Can you work these out from the model? Positions are in its coordinate system, mm. Face numbers are marked on the shaded views. A direction names the side the tool comes from. Give positions to 0.01 mm unless a question says otherwise; leave off trailing zeros. Order: outer loops, then holes, each group sorted by start corner. A loop starts at its lowest first (then second) coordinate and runs counter-clockwise, first axis right, second up. Notation, with made-up numbers: M 34.25,29 L 50.25,29 A18 cw 50.25,56 Z; hole C 22.5,15.25 d4. An arc over 180 degrees is marked long. Use one line per item in the form item = value. Start each with the question number.
1. I want a section at D-D, the plane z = -407.5. List the corners of the cut face in (x, y) for me, and give its area (3 significant figures).
2. I want a section at B-B, the plane x = -337.5. List the corners of the cut face in (y, z) for me, and give its area (3 significant figures).
3. I want a section at A-A, the plane z = -257. List the corners of the cut face in (x, y) for me, and give its area (3 significant figures).
4. We'd pull the mould along Y, two halves only. Please class the marked faces 1, 2 and 3: +Y half, -Y half, draft (parallel to the pull), parting line (faces both ways), or undercut.
5. Will these pins go through, and if not, where does the flat tip stop? P1, Ø7, axis at y = -237, z = -459, coming from the +X side; P2, Ø12, axis at x = 105.5, z = -649.5, coming from the +Y side; P3, Ø4, axis at y = -147, z = -600.5, coming from the +X side; P4, Ø6, axis at x = 309, y = -69, coming from the +Z side.
6. For the marked faces 4, 5 and 6, which set-ups out of +Z, -Z, +X, -X, +Y, -Y let a thin tool reach every point of the face, with its end or its side?
7. I need wall thicknesses on L1, parallel to Y at x = -5.5, z = -684.5; L2, parallel to Y at x = 99, z = -420.5; L3, parallel to X at y = 13, z = -487.5. Which ranges of each line are inside material? Lowest first, please.
```python
from build123d import *

# Parameters (mm, degrees)
F0_W      = 76.2
F0_H      = 76.2
F1_DEPTH  = 812.8
F2_DEPTH  = 736.6
F0_W_2    = 800.1
F0_H_2    = 482.6
F3_DEPTH  = 25.4
F4_W      = 355.6
F4_H      = 76.2
F5_DEPTH  = 101.6
F6_R      = 38.09999
F7_W      = 298.45
F7_H      = 533.4
F7_W_2    = 12.7
F7_H_2    = 127
F7_W_3    = 622.3
F7_H_3    = 101.6
F7_W_4    = 127
F7_H_4    = 12.7
F8_DEPTH  = 6.35
F9_DEPTH  = 12.7
F10_W     = 222.25
F10_H     = 482.6
F11_DEPTH = 25.4
F12_W     = 622.3
F12_H     = 304.8
F13_DEPTH = 635


# Not quite as in the source:
# - a fillet or chamfer is up to 0.001 mm smaller than in the source, because OpenCascade refuses the exact size


with BuildPart() as f1:
    # F0 (on Top) → F1 (new body)
    with BuildSketch(Plane.XY):
        with Locations((-349.25, 190.5)):
            Rectangle(F0_W, F0_H)
    extrude(amount=-F1_DEPTH)



with BuildPart() as f1b:
    # F0 (on Top) → F1, piece 2 (new body)
    with BuildSketch(Plane.XY):
        with Locations((-349.25, -190.5)):
            Rectangle(F0_W, F0_H)
    extrude(amount=-F1_DEPTH)


with BuildPart() as f1c:
    # F0 (on Top) → F1, piece 3 (new body)
    with BuildSketch(Plane.XY):
        with Locations((349.25, -190.5)):
            Rectangle(F0_W, F0_H)
    extrude(amount=-F1_DEPTH)


with BuildPart() as f1d:
    # F0 (on Top) → F1, piece 4 (new body)
    with BuildSketch(Plane.XY):
        with Locations((349.25, 190.5)):
            Rectangle(F0_W, F0_H)
    extrude(amount=-F1_DEPTH)


with BuildPart() as f1_1:
    add(f1.part)

    add(f1b.part)  # F2 merges F1b

    add(f1c.part)  # F2 merges F1c

    add(f1d.part)  # F2 merges F1d
    # F0 (on Top) → F2 (join)
    with BuildSketch(Plane.XY):
        with Locations((-349.25, 190.5)):
            Rectangle(F0_W, F0_H)
        Polygon((311.15, 152.4), (311.15, 228.6), (-311.15, 228.6), (-311.15, 152.4), (-387.35, 152.4), (-387.35, -152.4), (-311.15, -152.4), (-311.15, -228.6), (311.15, -228.6), (311.15, -152.4), (387.35, -152.4), (387.35, 152.4), align=None)
        with Locations((-349.25, -190.5)):
            Rectangle(F0_W, F0_H)
        with Locations((349.25, -190.5)):
            Rectangle(F0_W, F0_H)
        with Locations((349.25, 190.5)):
            Rectangle(F0_W, F0_H)
    extrude(amount=-F2_DEPTH)

    # F0 (on Top) → F3 (join)
    with BuildSketch(Plane.XY):
        Rectangle(F0_W_2, F0_H_2)
        Polygon((311.15, 228.6), (387.35, 228.6), (387.35, 152.4), (387.35, -152.4), (387.35, -228.6), (311.15, -228.6), (-311.15, -228.6), (-387.35, -228.6), (-387.35, -152.4), (-387.35, 152.4), (-387.35, 228.6), (-311.15, 228.6), align=None, mode=Mode.SUBTRACT)
    extrude(amount=-F3_DEPTH)

    # F4 (on face) → F5 (join)
    with BuildSketch(Plane.YZ.offset(387.35)):
        with Locations((0, -139.7)):
            Rectangle(F4_W, F4_H)
    extrude(amount=F5_DEPTH)

    # F6 (radius 38.1 in the source; OpenCascade refuses exactly that, so slightly less here)
    f6_edges = [f1_1.edges().sort_by_distance(p)[0] for p in [
        (488.95, 0, -101.6),
        (488.95, 0, -177.8),
    ]]
    fillet(f6_edges, radius=F6_R)

    # F7 (on face) → F8 (join)
    with BuildSketch(Plane.XZ.offset(228.6)):
        with Locations((161.925, -444.5)):
            Rectangle(F7_W, F7_H)
        with Locations((44.45, -444.5)):
            Rectangle(F7_W_2, F7_H_2, mode=Mode.SUBTRACT)
        with Locations((-161.925, -444.5)):
            Rectangle(F7_W, F7_H)
        with Locations((-44.45, -444.5)):
            Rectangle(F7_W_2, F7_H_2, mode=Mode.SUBTRACT)
        with Locations((0, -101.6)):
            Rectangle(F7_W_3, F7_H_3)
        with Locations((0, -101.6)):
            Rectangle(F7_W_4, F7_H_4, mode=Mode.SUBTRACT)
        with Locations((0, -101.6)):
            Rectangle(F7_W_4, F7_H_4)
        with Locations((44.45, -444.5)):
            Rectangle(F7_W_2, F7_H_2)
        with Locations((-44.45, -444.5)):
            Rectangle(F7_W_2, F7_H_2)
    extrude(amount=F8_DEPTH)

    # F7 (on face) → F9 (join)
    with BuildSketch(Plane.XZ.offset(228.6)):
        with Locations((0, -101.6)):
            Rectangle(F7_W_4, F7_H_4)
        with Locations((-44.45, -444.5)):
            Rectangle(F7_W_2, F7_H_2)
        with Locations((44.45, -444.5)):
            Rectangle(F7_W_2, F7_H_2)
    extrude(amount=F9_DEPTH)

    # F10 (on face) → F11 (join, through all)
    with BuildSketch(Plane.XY):
        with Locations((-511.175, 0)):
            Rectangle(F10_W, F10_H)
    extrude(amount=-F11_DEPTH)

    # F12 (on face) → F13 (cut)
    with BuildSketch(Plane(origin=(0, 0, -736.6), x_dir=(1, 0, 0), z_dir=(0, 0, -1))):
        Rectangle(F12_W, F12_H)
    extrude(amount=-F13_DEPTH, mode=Mode.SUBTRACT)


solid = f1_1.part
```
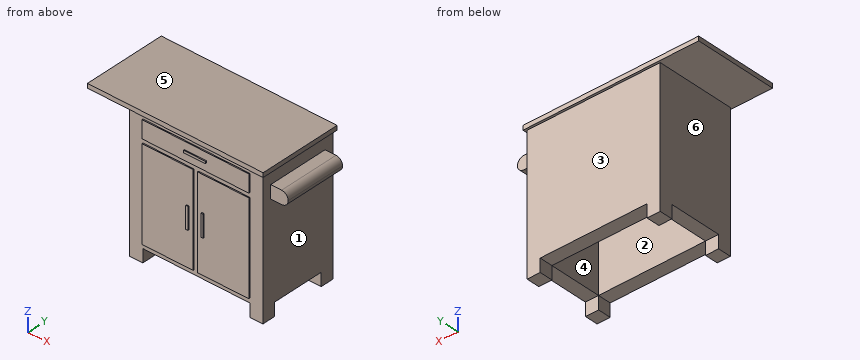
Check result:
q1.outline = M -387.35,-228.6 L -311.15,-228.6 L -311.15,-234.95 L -50.8,-234.95 L -50.8,-241.3 L -38.1,-241.3 L -38.1,-234.95 L -12.7,-234.95 L -12.7,-228.6 L 12.7,-228.6 L 12.7,-234.95 L 38.1,-234.95 L 38.1,-241.3 L 50.8,-241.3 L 50.8,-234.95 L 311.15,-234.95 L 311.15,-228.6 L 387.35,-228.6 L 387.35,228.6 L -387.35,228.6 Z; hole M -311.15,-152.4 L 311.15,-152.4 L 311.15,152.4 L -311.15,152.4 Z
q1.area = 168,000 mm2
q2.outline = M -241.3,-25.4 L -228.6,-25.4 L -228.6,-812.8 L -152.4,-812.8 L -152.4,-736.6 L 152.4,-736.6 L 152.4,-812.8 L 228.6,-812.8 L 228.6,-25.4 L 241.3,-25.4 L 241.3,0 L -241.3,0 Z
q2.area = 349,000 mm2
q3.outline = M -387.35,-228.6 L -311.15,-228.6 L -311.15,-234.95 L -12.7,-234.95 L -12.7,-228.6 L 12.7,-228.6 L 12.7,-234.95 L 311.15,-234.95 L 311.15,-228.6 L 387.35,-228.6 L 387.35,228.6 L -387.35,228.6 Z; hole M -311.15,-152.4 L 311.15,-152.4 L 311.15,152.4 L -311.15,152.4 Z
q3.area = 168,000 mm2
q4.face_1 = draft
q4.face_2 = undercut
q4.face_3 = +Y half
q5.P1 = 311.15
q5.P2 = 228.6
q5.P3 = 387.35
q5.P4 = 0
q6.face_4 = -Z
q6.face_5 = +Z, +X, -X, +Y, -Y
q6.face_6 = -Z, -X, +Y, -Y
q7.L1 = -228.6 to -152.4, 152.4 to 228.6
q7.L2 = -234.95 to -152.4, 152.4 to 228.6
q7.L3 = -387.35 to -311.15, 311.15 to 387.35
